Solid Edge part; units mm, degrees
sketch "Sketch1" plane through (0, 0, 0) normal (0, 0, 1) x (1, 0, 0)
  circle A0 centre (0, 0) radius 7.5
extrude "Protrusion1" add sketch "Sketch1" along normal blind 30
sketch "Sketch2" plane through (0, 0, 30) normal (0, 0, 1) x (1, 0, 0)
  circle A0 centre (0, 0) radius 2
extrude "ExtrudedCutout_1" cut sketch "Sketch2" against normal blind 15
sketch "Sketch3" plane through (0, 0, 0) normal (0, 0, -1) x (1, 0, 0)
  line L0 (-1.9999, -1.5001) -> (-1.9999, 1.5001)
  arc A0 (-1.9999, 1.5001) -> (-1.9999, -1.5001) centre (0, 0) cw
extrude "Cutout1" cut sketch "Sketch3" against normal up to vertex (15 mm away)
sketch "Sketch4" plane through (-7.5, 0, 15) normal (-1, 0, 0) x (0, 0, -1)
  line L0 (5.4123, 2.75) -> (3.8246, 0)
  line L1 (3.8246, 0) -> (5.4123, -2.75)
  line L2 (5.4123, -2.75) -> (8.5877, -2.75)
  line L3 (8.5877, -2.75) -> (10.1754, 0)
  line L4 (10.1754, 0) -> (8.5877, 2.75)
  line L5 (8.5877, 2.75) -> (5.4123, 2.75)
  line L6 (-8.5877, 2.75) -> (-10.1754, 0)
  line L7 (-10.1754, 0) -> (-8.5877, -2.75)
  line L8 (-8.5877, -2.75) -> (-5.4123, -2.75)
  line L9 (-5.4123, -2.75) -> (-3.8246, 0)
  line L10 (-3.8246, 0) -> (-5.4123, 2.75)
  line L11 (-5.4123, 2.75) -> (-8.5877, 2.75)
extrude "ExtrudedCutout_3" cut sketch "Sketch4" against normal blind 3
sketch "Sketch5" plane through (-7.5, 0, 15) normal (-1, 0, 0) x (0, 0, -1)
  circle A0 centre (-7, 0) radius 1.35
  circle A1 centre (7, 0) radius 1.35
extrude "Cutout2" cut sketch "Sketch5" against normal up to next
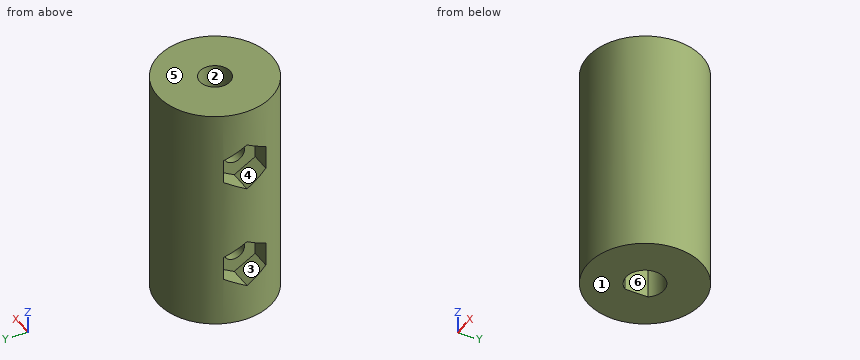
For this review, take the finished solid that the model builds, in its own axes (mm). Face numbers are marked on the shaded views. A direction names the side the tool comes from. Round coordinates to 2 decimals unless told otherwise and drop trailing zeros. Write each loop counter-clockwise with the first axis right and the second up, starting at its lowest first coordinate (ties: lowest second). Pieces come first, ordered by that corner, then holes. Notation, with made-up numbers: (-33, -7.5) - (-17, -7.5) arc R23 cw to (-17, 31.5) - close; hole circle Ø11 at (-8, 53.25). An arc over 180 degrees is marked (long way). Write each question's results on one line, items separated by ' | '.
Item 1: Take a section at C-C on z = 8. State the section outline as (x, y) points.
Calculated:
outline: (-6.98, -2.75) arc R7.5 ccw (long way) to (-6.98, 2.75) - (-4.5, 2.75) - (-4.5, 1.35) - (-2, 1.35) - (-2, 1.5) arc R2.5 cw (long way) to (-2, -1.5) - (-2, -1.35) - (-4.5, -1.35) - (-4.5, -2.75) - close
Item 2: Take a section at A-A on x = 0. State the section outline as (y, z) points, then the cut area to 3 significant figures.
Calculated:
outline: (-7.5, 0) - (-2.5, 0) - (-2.5, 15) - (-2, 15) - (-2, 30) - (-7.5, 30) - close; (2, 15) - (2.5, 15) - (2.5, 0) - (7.5, 0) - (7.5, 30) - (2, 30) - close | area: 315 mm^2
Item 3: Take a section at B-B on z = 4. State the section outline as (x, y) points.
Calculated:
outline: circle Ø15 at (0, 0); hole (-2, -1.5) arc R2.5 ccw (long way) to (-2, 1.5) - close
Item 4: Draft analysis for pull direction Z (two halves, no side actions). For the marked faces 1, 2 and 3, state which applies: pulls with the +Z half, pulls with the -Z half, needs draft (parallel to the pull), parting line crosses it, or undercut.
Calculated:
face 1: pulls with the -Z half | face 2: needs draft | face 3: undercut
Item 5: For pin 1 (2.5 mm diameter, centred on x = -6, z = 21.5, fed in from +Y); pin 2 (0.7 mm diameter, centred on x = -5.5, z = 8.5, fed in from +Y); pin 3 (6 mm diameter, centred on x = -5, z = 6, fed in from -Y), all flat-tipped, find the tip position at first contact; note any pin that passes through.
Calculated:
pin 1: stops at y = 5.8 | pin 2: stops at y = 5.45 | pin 3: stops at y = -7.23
Item 6: Take a section at D-D on y = 6. State the section outline as (x, z) points.
Calculated:
outline: (-4.5, 0) - (4.5, 0) - (4.5, 30) - (-4.5, 30) - close
Item 7: For the marked faces 4, 5 and 6, list the 3-axis set-ups (+Z, -Z, +X, -X, +Y, -Y) from which the entire face can be reached by the end or side of a thin tool; tool diameter is ignored.
Calculated:
face 4: -X | face 5: +Z, +X, -X, +Y, -Y | face 6: -Z
Item 8: To check wall thickness, follow line 1 along X through (y, z) = (0, 18); line 2 along X through (y, z) = (0, 11.5). State the ranges of each line that lie inside material, in increasing order. Write a range as from..to.
Calculated:
line 1: x = -7.5..-2, 2..7.5 | line 2: x = -7.5..-2, 2.5..7.5
